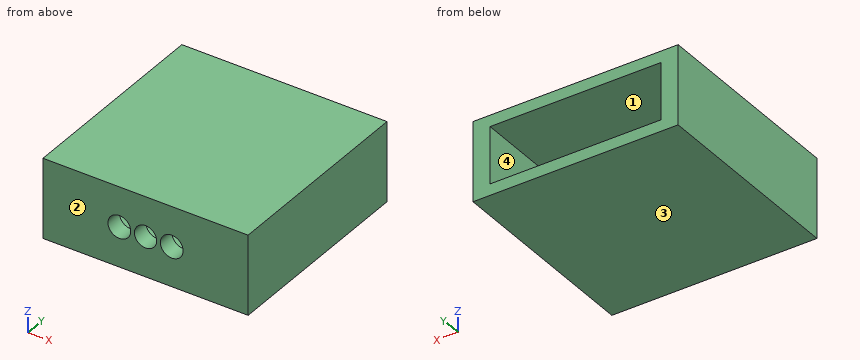
```python
from build123d import *

# Parameters (mm, degrees)
SKETCH1_W           = 45.72
SKETCH1_H           = 17.78
BOSS_EXTRUDE1_DEPTH = 45.72
SKETCH2_W           = 38.1
SKETCH2_H           = 12.7
CUT_EXTRUDE1_DEPTH  = 41.91
SKETCH3_R           = 2.4765
SKETCH3_R_2         = 2.54
CUT_EXTRUDE2_DEPTH  = 46.72


with BuildPart() as part:
    # Sketch1 → Boss-Extrude1 (new body)
    with BuildSketch(Plane(origin=(0, 0, 0), x_dir=(1, 0, 0), z_dir=(0, 1, 0))):
        with Locations((22.86, 8.89)):
            Rectangle(SKETCH1_W, SKETCH1_H)
    extrude(amount=BOSS_EXTRUDE1_DEPTH)

    # Sketch2 → Cut-Extrude1 (cut)
    with BuildSketch(Plane(origin=(0, 45.72, 0), x_dir=(1, 0, 0), z_dir=(0, 1, 0))):
        with Locations((22.86, 8.89)):
            Rectangle(SKETCH2_W, SKETCH2_H)
    extrude(amount=-CUT_EXTRUDE1_DEPTH, mode=Mode.SUBTRACT)

    # Sketch3 → Cut-Extrude2 (cut, through all)
    with BuildSketch(Plane(origin=(0, 0, 0), x_dir=(1, 0, 0), z_dir=(0, 1, 0))):
        with Locations((22.86, 8.89)):
            Circle(SKETCH3_R)
        with Locations((17.018, 8.89)):
            Circle(SKETCH3_R_2)
        with Locations((28.702, 8.89)):
            Circle(SKETCH3_R_2)
    extrude(amount=CUT_EXTRUDE2_DEPTH, mode=Mode.SUBTRACT)


solid = part.part
```
Read the model definition and answer for the solid it produces. Units are mm, in the model's axes. Face numbers are marked on the shaded views. Give positions to 0.01 mm unless a question says otherwise; leave off trailing zeros. Order: outer loops, then holes, each group sorted by start corner. A loop starts at its lowest first (then second) coordinate and runs counter-clockwise, first axis right, second up.
(1) Given pin 1 (4 mm diameter, centred on x = 22.86, z = -8.89, fed in from -Y), flat-ended and moving along its own axis, determine where the tip first touches the part or whether it passes through.
(2) Find section B-B (x = 22.86). Give the vertices of the cut face in (y, z), plus the area to 3 significant figures.
(3) Straight lines are drawn through the part: L1, parallel to X at y = 1.55, z = -8.89; L2, parallel to Z at x = 30, y = 31; L3, parallel to X at y = 10.5, z = -10.5. For each, find the intervals that lie inside material, in ascending order.
(4) For a pull along Z with two mould halves and no side action, classify the marked faces 1, 2, 3 and 4 as released by +Z, released by -Z, zero draft, split by the parting line, or undercut.
(5) Find section D-D (z = -5.25). Give the vertices of the cut face in (x, y).
(6) Find section A-A (z = -8.89). Give the vertices of the cut face in (x, y).
(7) Find section C-C (y = 16.5). Give the vertices of the cut face in (x, z), plus the area to 3 significant figures.
Result sheet:
1. pin 1: passes through
2. outline: (0, -17.78) - (45.72, -17.78) - (45.72, -15.24) - (3.81, -15.24) - (3.81, -11.37) - (0, -11.37) - close; (0, -6.41) - (3.81, -6.41) - (3.81, -2.54) - (45.72, -2.54) - (45.72, 0) - (0, 0) - close
2. area: 262 mm2
3. L1: x = 0 to 14.48, 19.56 to 20.38, 25.34 to 26.16, 31.24 to 45.72
3. L2: z = -17.78 to -15.24, -2.54 to 0
3. L3: x = 0 to 3.81, 41.91 to 45.72
4. face 1: undercut
4. face 2: zero draft
4. face 3: released by -Z
4. face 4: undercut
5. outline: (0, 0) - (45.72, 0) - (45.72, 45.72) - (41.91, 45.72) - (41.91, 3.81) - (3.81, 3.81) - (3.81, 45.72) - (0, 45.72) - close
6. outline: (0, 0) - (14.48, 0) - (14.48, 3.81) - (3.81, 3.81) - (3.81, 45.72) - (0, 45.72) - close; (19.56, 0) - (20.38, 0) - (20.38, 3.81) - (19.56, 3.81) - close; (25.34, 0) - (26.16, 0) - (26.16, 3.81) - (25.34, 3.81) - close; (31.24, 0) - (45.72, 0) - (45.72, 45.72) - (41.91, 45.72) - (41.91, 3.81) - (31.24, 3.81) - close
7. outline: (0, -17.78) - (45.72, -17.78) - (45.72, 0) - (0, 0) - close; hole (3.81, -15.24) - (41.91, -15.24) - (41.91, -2.54) - (3.81, -2.54) - close
7. area: 329 mm2
